```python
from build123d import *

# Parameters (mm, degrees)
BOSS_EXTRUDE1_DEPTH = 3.3
BOSS_EXTRUDE2_DEPTH = 13.6
BOSS_EXTRUDE3_DEPTH = 3.3


with BuildPart() as part:
    # Sketch1 → Boss-Extrude1 (new body)
    with BuildSketch(Plane(origin=(0, 0, 0), x_dir=(1, 0, 0), z_dir=(0, 1, 0))):
        Polygon((0, 0), (27.8, 0), (27.8, 4), (23.8, 4), (4, 23.8), (4, 27.8), (0, 27.8), align=None)
    extrude(amount=BOSS_EXTRUDE1_DEPTH)

    # Sketch2 → Boss-Extrude2 (add)
    with BuildSketch(Plane.XZ):
        Polygon((0, 0), (27.8, 0), (27.8, -3.3), (3.3, -3.3), (3.3, -27.8), (0, -27.8), align=None)
    extrude(amount=BOSS_EXTRUDE2_DEPTH)

    # Sketch3 → Boss-Extrude3 (add)
    with BuildSketch(Plane.XZ.offset(13.6)):
        Polygon((27.8, -3.3), (27.8, 0), (0, 0), (0, -27.8), (3.3, -27.8), (4, -27.8), (4, -23.8), (23.8, -4), (27.8, -4), align=None)
    extrude(amount=BOSS_EXTRUDE3_DEPTH)


solid = part.part
```
Can you work these out from the model? Positions are in its coordinate system, mm. A direction names the side the tool comes from. Give positions to 0.01 mm unless a question says otherwise; leave off trailing zeros. Write each loop counter-clockwise with the first axis right and the second up, starting at its lowest first coordinate (ties: lowest second). Pieces come first, ordered by that corner, then holes. Notation, with made-up numbers: (-5, 34.5) - (21, 34.5) arc R16 cw to (21, 59.5) - close; hole circle Ø8 at (79, 46.5). An arc over 180 degrees is marked (long way). Write item = value, one per line. Start each with the question number.
1. On a 3-axis mill with a long thin cutter (end or side, diameter ignored), from which of +Z, -Z, +X, -X, +Y, -Y can I reach the whole of each face in a straight line? I mean faces 1 (the face through (4, -15, -26)), 2 (the face through (10, 0, -11)), 3 (the face through (27.8, -7, -2)). Say none if no direction works.
2. Thinking about a two-plate mould opening in Y: for faces 4 (the face through (8, 3.3, -8)), 5 (the face through (2, -7, -27.8)), 6 (the face through (10, -13.6, -10)), which applies, released by +Y, released by -Y, zero draft, split by the parting line, or undercut?
3. Imagine slicing it at A-A (x = 14.75). Please give me the cut outline in (y, z).
4. For pin 1 (5 mm diameter, centred on x = 6, y = -1, fed in from -Z); pin 2 (12 mm diameter, centred on x = 17.5, y = -7, fed in from -Z); pin 3 (1.6 mm diameter, centred on y = -15.5, z = -26, fed in from +X); pin 4 (1.5 mm diameter, centred on x = 13.5, y = -14, fed in from -Z), each with a flat end and sliding along its axis, tell me the tip position at first contact or that it passes through.
5. Imagine slicing it at B-B (z = -24.75). Please give me the cut outline in (x, y), and give its area (3 significant figures).
6. Please list where these lines run through material, in increasing order: line 1 (Y direction, x = 5.25, z = -11.75); line 2 (Z direction, x = 8.5, y = -2.5); line 3 (X direction, y = -3.5, z = -20.75).
7. Imagine slicing it at C-C (y = -10.5). Please give me the cut outline in (x, z).
Worked answers:
q1.face_1 = -Z, +X, +Y, -Y
q1.face_2 = -Z, +X
q1.face_3 = +Z, -Z, +X, +Y, -Y
q2.face_4 = released by +Y
q2.face_5 = zero draft
q2.face_6 = undercut
q3.outline = (-16.9, -13.05) - (-13.6, -13.05) - (-13.6, -3.3) - (0, -3.3) - (0, -13.05) - (3.3, -13.05) - (3.3, 0) - (-16.9, 0) - close
q4.pin_1 = -27.8
q4.pin_2 = -3.3
q4.pin_3 = 4
q4.pin_4 = -15.05
q5.outline = (0, -16.9) - (4, -16.9) - (4, -13.6) - (3.3, -13.6) - (3.3, 0) - (4, 0) - (4, 3.3) - (0, 3.3) - close
q5.area = 71.3 mm2
q6.line_1 = -16.9 to -13.6, 0 to 3.3
q6.line_2 = -3.3 to 0
q6.line_3 = 0 to 3.3
q7.outline = (0, -27.8) - (3.3, -27.8) - (3.3, -3.3) - (27.8, -3.3) - (27.8, 0) - (0, 0) - close
